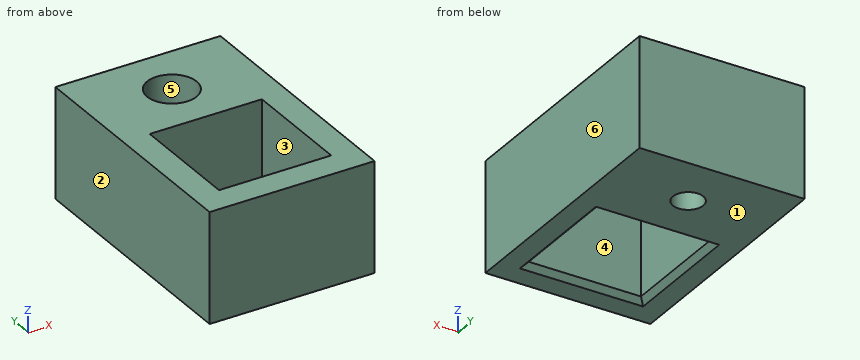
from build123d import *

# Parameters (mm, degrees)
SKETCH_W         = 30
SKETCH_H         = 45.4
SKETCH_W_2       = 20.4
SKETCH_H_2       = 20.4
PAD_DEPTH        = 20
HOLE_D           = 5.5
HOLE_CBORE_D     = 9
HOLE_CBORE_DEPTH = 15
CHAMFER_SIZE     = 1


with BuildPart() as part:
    # Sketch → Pad (new body)
    with BuildSketch(Plane.XY):
        with Locations((15, 22.7)):
            Rectangle(SKETCH_W, SKETCH_H)
        with Locations((15, 15.2)):
            Rectangle(SKETCH_W_2, SKETCH_H_2, mode=Mode.SUBTRACT)
    extrude(amount=PAD_DEPTH)

    # Hole (through all)
    with Locations(Plane.XY.offset(20)):
        with Locations((15, 35.4)):
            CounterBoreHole(HOLE_D / 2, HOLE_CBORE_D / 2, HOLE_CBORE_DEPTH)

    # Chamfer
    chamfer_edges = [part.edges().sort_by_distance(p)[0] for p in [
        (15, 25.4, 0),
        (25.2, 15.2, 0),
        (4.8, 15.2, 0),
        (15, 5, 0),
    ]]
    chamfer(chamfer_edges, length=CHAMFER_SIZE)


solid = part.part
Work out the finished part from the listing and answer in its coordinate system (mm). Face numbers are marked on the shaded views. A direction names the side the tool comes from. Coordinates: 2 decimals unless noted, no trailing zeros. Write each loop counter-clockwise with the first axis right and the second up, starting at its lowest first coordinate (ties: lowest second). Pieces come first, ordered by that corner, then holes. Notation, with made-up numbers: M 56,56.25 L 70,56.25 A27 cw 70,77.25 Z; hole C 51,8 d3. An arc over 180 degrees is marked long. Use one line per item in the form item = value. Start each with the question number.
1. A tool of negligible diameter and unlimited length cuts with its end or side. For the marked faces 4, 5 and 6, from which of +Z, -Z, +X, -X, +Y, -Y can it reach the whole face along a straight path? Write none if from no direction.
2. The part is cut by section A-A (y = 35.4). Give the vertices of the cut face in (x, z), plus the area to 4 significant figures.
3. This flat-tipped pin is pushed along its axis until it touches: P1, Ø7, axis at x = 15, y = 35.4, coming from the +Z side. Where does it stop, or does it pass through?
4. The part is cut by section D-D (z = 9.5). Give the vertices of the cut face in (x, y).
5. The mould has two halves that part along X. Classify the marked faces 1, 2 and 3: released by +X, released by -X, zero draft, split by the parting line, or undercut.
6. The part is cut by section C-C (x = 15). Give the vertices of the cut face in (y, z).
7. Straight lines are drawn through the part: probe 1 along Y at (x, z) = (15, 3.85); probe 2 along Y at (x, z) = (15, 12.75); probe 3 along Y at (x, z) = (24.25, 3). For each, find the intervals that lie inside material, in ascending order. Write a range as from..to.
8. The part is cut by section B-B (x = 20). Give the vertices of the cut face in (y, z).
Evaluation:
q1.face_4 = +Z, -Z
q1.face_5 = +Z
q1.face_6 = +Z, -Z, +X, +Y, -Y
q2.outline = M 0,0 L 12.25,0 L 12.25,5 L 10.5,5 L 10.5,20 L 0,20 Z; M 17.75,0 L 30,0 L 30,20 L 19.5,20 L 19.5,5 L 17.75,5 Z
q2.area = 437.5 mm^2
q3.P1 = 5
q4.outline = M 0,0 L 30,0 L 30,45.4 L 0,45.4 Z; hole M 4.8,5 L 25.2,5 L 25.2,25.4 L 4.8,25.4 Z; hole C 15,35.4 d9
q5.face_1 = zero draft
q5.face_2 = released by -X
q5.face_3 = undercut
q6.outline = M 0,0 L 4,0 L 5,1 L 5,20 L 0,20 Z; M 25.4,1 L 26.4,0 L 32.65,0 L 32.65,5 L 30.9,5 L 30.9,20 L 25.4,20 Z; M 38.15,0 L 45.4,0 L 45.4,20 L 39.9,20 L 39.9,5 L 38.15,5 Z
q7.probe_1 = 0..5, 25.4..32.65, 38.15..45.4
q7.probe_2 = 0..5, 25.4..30.9, 39.9..45.4
q7.probe_3 = 0..5, 25.4..45.4
q8.outline = M 0,0 L 4,0 L 5,1 L 5,20 L 0,20 Z; M 25.4,1 L 26.4,0 L 45.4,0 L 45.4,20 L 25.4,20 Z
